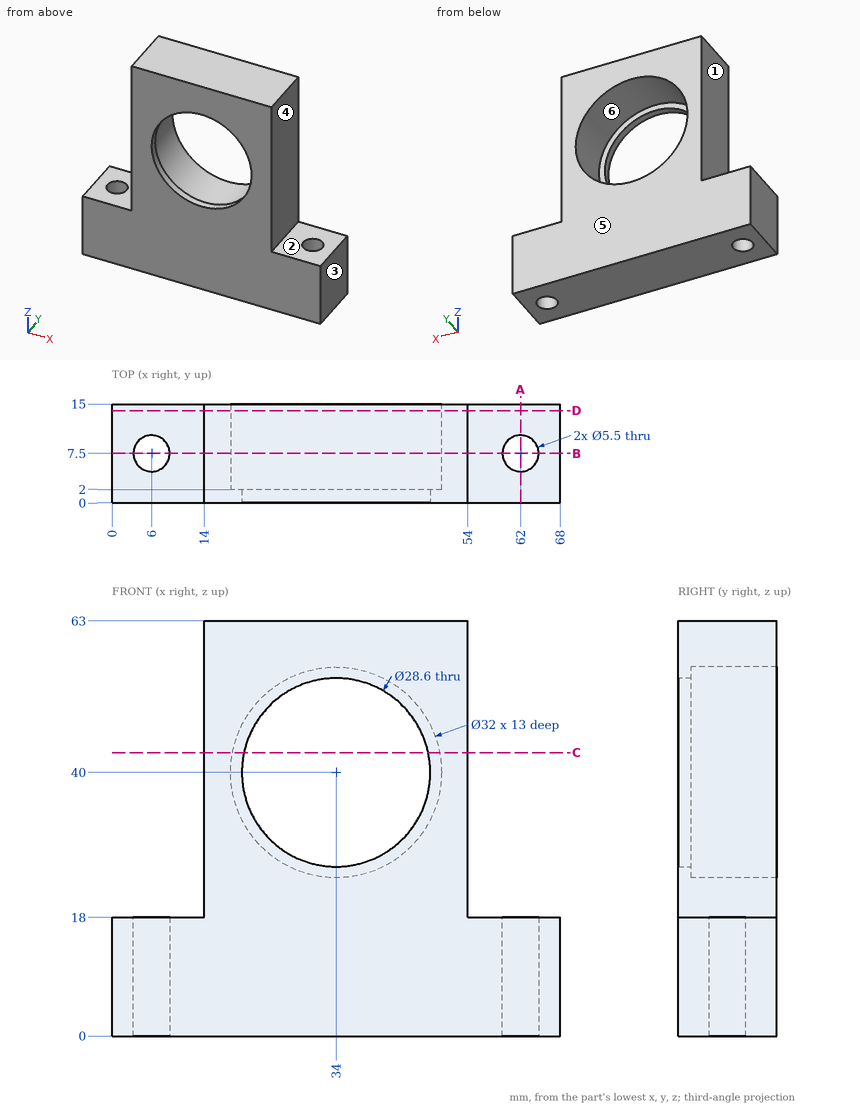
The figure shows three views and two pictorial views of one solid part (mm, origin at its lowest corner). Answer the questions. A direction names the side the tool comes from. Give positions to 0.01 mm unless a question says otherwise; leave off trailing zeros. Order: outer loops, then holes, each group sorted by start corner. A loop starts at its lowest first (then second) coordinate and runs counter-clockwise, first axis right, second up. Notation, with made-up numbers: (67.25, -23) - (72.25, -23) arc R25 ccw to (72.25, 4) - close; hole circle Ø6 at (11.5, 36). An arc over 180 degrees is marked (long way). Answer as CSV lines item,"result".
Q1. Which of the six approach directions +Z, -Z, +X, -X, +Y, -Y give full straight-line access (tool end or side, diameter ignored) to the marked faces 1, 2 and 3?
Answer key:
face 1,"+Z, -X, +Y, -Y"
face 2,"+Z, +X, +Y, -Y"
face 3,"+Z, -Z, +X, +Y, -Y"
Q2. Each of these flat-tipped pins is pushed along its axis until it touches: pin 1 Ø1 at (y, z) = (7, 18) entering from -X; pin 2 Ø9 at (x, y) = (62, 7.5) entering from +Z; pin 3 Ø2 at (y, z) = (3, 22.5) entering from +X. Where does it stop, or does it pass through?
Answer key:
pin 1,"stops at x = 0"
pin 2,"stops at z = 18"
pin 3,"stops at x = 54"
Q3. Determine the mould class of the marked faces 4, 5 and 6 for opening direction X: pulls with the +X half, pulls with the -X half, needs draft (parallel to the pull), parting line crosses it, or undercut.
Answer key:
face 4,"pulls with the +X half"
face 5,"needs draft"
face 6,"undercut"
Q4. Straight lines are drawn through the part: L1, parallel to Y at x = 6, z = 6; L2, parallel to Z at x = 57.5, y = 12.5; L3, parallel to X at y = 2.75, z = 60. For each, find the intervals that lie inside material, in ascending order.
Answer key:
L1,"y = 0 to 4.75, 10.25 to 15"
L2,"z = 0 to 18"
L3,"x = 14 to 54"
Q5. A cutting plane is placed at B-B, the plane y = 7.5. Determine the outline of the cut face in (x, z).
Answer key:
outline,"(0, 0) - (3.25, 0) - (3.25, 18) - (0, 18) - close; (8.75, 0) - (59.25, 0) - (59.25, 18) - (54, 18) - (54, 63) - (14, 63) - (14, 18) - (8.75, 18) - close; (64.75, 0) - (68, 0) - (68, 18) - (64.75, 18) - close; hole circle Ø32 at (34, 40)"
Q6. A cutting plane is placed at C-C, the plane z = 43. Determine the outline of the cut face in (x, y).
Answer key:
outline,"(14, 0) - (20.02, 0) - (20.02, 2) - (18.28, 2) - (18.28, 15) - (14, 15) - close; (47.98, 0) - (54, 0) - (54, 15) - (49.72, 15) - (49.72, 2) - (47.98, 2) - close"
Q7. A cutting plane is placed at A-A, the plane x = 62. Determine the outline of the cut face in (y, z).
Answer key:
outline,"(0, 0) - (4.75, 0) - (4.75, 18) - (0, 18) - close; (10.25, 0) - (15, 0) - (15, 18) - (10.25, 18) - close"
Q8. A cutting plane is placed at D-D, the plane y = 14. Determine the outline of the cut face in (x, z).
Answer key:
outline,"(0, 0) - (68, 0) - (68, 18) - (54, 18) - (54, 63) - (14, 63) - (14, 18) - (0, 18) - close; hole circle Ø32 at (34, 40)"
